Geometry check sheet. Reference: the model listing, model coordinates, mm. Give positions to 0.01 mm unless a question says otherwise; leave off trailing zeros. Write each loop counter-clockwise with the first axis right and the second up, starting at its lowest first coordinate (ties: lowest second). Pieces come first, ordered by that corner, then holes. Notation, with made-up numbers: (88, -15.5) - (143, -15.5) arc R9 ccw to (143, 0.5) - close; hole circle Ø8 at (6, 23.5). An arc over 180 degrees is marked (long way). Write item = value, one per line. Start each with the question number.
(1) Section check C-C, the plane x = 1.1. Enter the section's corners in (y, z).
(2) Thickness scan on L1, parallel to Z at x = 0.8, y = 0; L2, parallel to Y at x = 2.05, z = -6.2; L3, parallel to Y at x = 0.8, z = 0. Record the ranges inside material, lowest first.
(3) Section check B-B, the plane y = 1.5. Enter the section's corners in (x, z), plus the area to 3 significant figures.
(4) Depth check by flat-ended pin: pin 1 Ø3 at (y, z) = (-6.2, -6.2) entering from +X; pin 2 Ø2 at (y, z) = (-1, 1.5) entering from +X. Enter the tip coordinate at first touch or a pass-through.
(5) Section check D-D, the plane z = -6.2. Enter the section's corners in (x, y), plus the area to 3 significant figures.
(6) Section check A-A, the plane z = 0. Enter the section's corners in (x, y), plus the area to 3 significant figures.
Autodesk Inventor part; units mm, degrees
ref_plane "YZ Plane" through (0, 0, 0) normal (1, 0, 0) x (0, 1, 0)
ref_plane "XZ Plane" through (0, 0, 0) normal (0, 1, 0) x (-1, 0, 0)
ref_plane "XY Plane" through (0, 0, 0) normal (0, 0, 1) x (1, 0, 0)
sketch "Эскиз1" plane through (0, 0, 0) normal (1, 0, 0) x (0, 1, 0)
  circle A0 centre (35.2311, -22.6062) radius 9.3
  circle A1 centre (0, -38.8201) radius 6.1
  circle A2 centre (0, 0) radius 4.85
  circle A3 centre (35.8147, -49.5529) radius 3.55
  line L0 (6.0968, -38.6237) -> (4.8475, 0.1562)
  line L1 (-4.8475, 0.1562) -> (-6.0968, -38.6237)
  line L2 (0, 0) -> (0, -38.8201) construction
  circle A4 centre (0, -38.8201) radius 2
  circle A5 centre (0, 0) radius 2
  circle A6 centre (0, -38.8201) radius 15 construction
  circle A7 centre (0, 0) radius 14 construction
  circle A8 centre (0, -38.8201) radius 7
  circle A9 centre (0, 0) radius 7
  line L3 (6.9463, -39.6857) -> (11.7094, -1.459)
  line L4 (-6.9463, -39.6857) -> (-11.7094, -1.459)
  circle A10 centre (0, 0) radius 8.8
  circle A11 centre (0, 0) radius 11.8
  point P0 (-7, 0)
  point P1 (-6.9463, -39.6857)
  point P2 (-11.7094, -1.459)
  dimension "d27" = 14
  dimension "d0" = 18.6
  dimension "d1" = 12.2
  dimension "d2" = 9.7
  dimension "d3" = 7.1
  dimension "d8" = 38.8201
  dimension "d13" = 38.8
  dimension "d14" = 38.8
  dimension "d23" = 4
  dimension "d24" = 4
  dimension "d25" = 30
  dimension "d26" = 28
  dimension "d28" = 14
  dimension "d31" = 17.6
  dimension "d32" = 3
extrude "Выдавливание4" add sketch "Эскиз1" along normal blind 3 contours A1 | A1 L0 A8 L1 | A1 L1 A8 L0 | A8 L1 A11 L0 | L0 A11 L3 A8 | A8 L4 A11 L1 | A11 L1 A10 L0 | L0 A10 L1 A11 | A10 L1 A9 L0 | L0 A9 L1 A10 | A9 L1 A2 L0 | L0 A2 L1 A9 | A2
sketch "Эскиз4" plane through (0, 0, 0) normal (-1, 0, 0) x (0, 0, 1)
  circle A0 centre (-6.2, 6.2) radius 1.25
  circle A1 centre (0, 0) radius 2 construction
  circle A2 centre (-38.8201, 0) radius 2 construction
  arc A3 (-1.459, -11.7094) -> (-1.459, 11.7094) centre (0, 0) ccw construction
  line L0 (-39.6857, 6.9463) -> (-1.459, 11.7094) construction
  arc A4 (-39.6857, 6.9463) -> (-39.6857, -6.9463) centre (-38.8201, 0) ccw construction
  line L1 (-1.459, -11.7094) -> (-39.6857, -6.9463) construction
  line L2 (0, 0) -> (0, 11.8) construction
  arc A5 (-1.459, -11.7094) -> (-1.459, 11.7094) centre (0, 0) ccw construction
  line L3 (0, 0) -> (11.8, 0) construction
  circle A6 centre (6.2, 6.2) radius 1.25
  circle A7 centre (-6.2, -6.2) radius 1.25
  circle A8 centre (6.2, -6.2) radius 1.25
  dimension "d33" = 2.5
  dimension "d34" = 12.4
  dimension "d35" = 12.4
extrude "Выдавливание5" cut sketch "Эскиз4" against normal blind 3
sketch "Эскиз5" plane through (3, 0, 0) normal (1, 0, 0) x (0, 0, -1)
  circle A0 centre (0, 0) radius 3.5
  dimension "d38" = 7
extrude "Выдавливание6" cut sketch "Эскиз5" against normal blind 1
properties part number "wall"
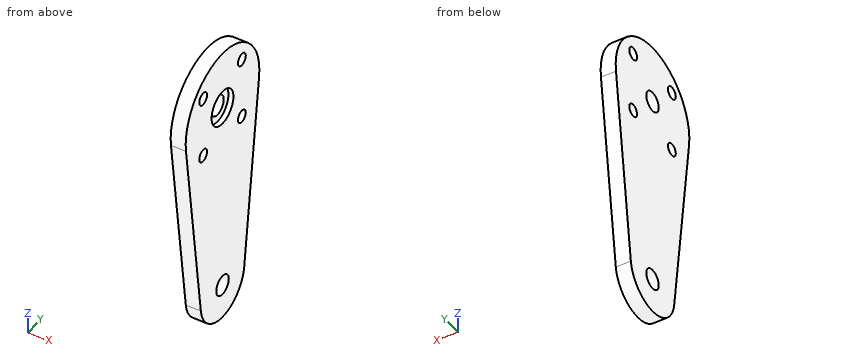
Model answer:
q1.outline = (-11.71, -1.46) - (-6.95, -39.69) arc R7 ccw to (6.95, -39.69) - (11.71, -1.46) arc R11.8 ccw (long way) to start; hole circle Ø2.5 at (-6.2, -6.2); hole circle Ø2.5 at (-6.2, 6.2); hole circle Ø4 at (0, -38.82); hole circle Ø4 at (0, 0); hole circle Ø2.5 at (6.2, -6.2); hole circle Ø2.5 at (6.2, 6.2)
q2.L1 = -45.82 to -40.82, -36.82 to -2, 2 to 11.8
q2.L2 = -11.12 to -7.45, -4.95 to 4.95, 7.45 to 11.12
q2.L3 = -11.8 to -2, 2 to 11.8
q3.outline = (0, -45.66) - (3, -45.66) - (3, -40.14) - (0, -40.14) - close; (0, -37.5) - (3, -37.5) - (3, -3.16) - (2, -3.16) - (2, -1.32) - (0, -1.32) - close; (0, 1.32) - (2, 1.32) - (2, 3.16) - (3, 3.16) - (3, 11.7) - (0, 11.7) - close
q3.area = 153 mm²
q4.pin_1 = 3
q4.pin_2 = 2
q5.outline = (0, -11.12) - (3, -11.12) - (3, -7.45) - (0, -7.45) - close; (0, -4.95) - (3, -4.95) - (3, 4.95) - (0, 4.95) - close; (0, 7.45) - (3, 7.45) - (3, 11.12) - (0, 11.12) - close
q5.area = 51.7 mm²
q6.outline = (0, -11.8) - (3, -11.8) - (3, -3.5) - (2, -3.5) - (2, -2) - (0, -2) - close; (0, 2) - (2, 2) - (2, 3.5) - (3, 3.5) - (3, 11.8) - (0, 11.8) - close
q6.area = 55.8 mm²
